Check sheet for the modelled part. Datum: model origin and axes. Units: mm. Round coordinates to 2 decimals unless told otherwise and drop trailing zeros. Order: outer loops, then holes, each group sorted by start corner. A loop starts at its lowest first (then second) coordinate and runs counter-clockwise, first axis right, second up. Notation, with made-up numbers: (75, 71.5) -> (121, 71.5) arc R13 ccw to (121, 93.5) -> close; hole circle Ø4 at (-34.5, 26). An arc over 180 degrees is marked (long way). Answer as CSV lines item,"result". Start each with the question number.
from build123d import *

# Parameters (mm, degrees)
SKETCH1_R           = 48.5
SKETCH1_R_2         = 4.7625
BOSS_EXTRUDE1_DEPTH = 10
CUT_EXTRUDE1_DEPTH  = 5000
SKETCH3_R           = 4.7625
CUT_EXTRUDE2_DEPTH  = 5000


with BuildPart() as part:
    # Sketch1 → Boss-Extrude1 (new body)
    with BuildSketch(Plane(origin=(0, 0, 0), x_dir=(1, 0, 0), z_dir=(0, 1, 0))):
        Polygon((205, 610), (-205, 610), (-305, 510), (-305, 100), (-205, 0), (205, 0), (305, 100), (305, 510), align=None)
        with Locations((-167.82128445, 168.589357775)):
            Circle(SKETCH1_R, mode=Mode.SUBTRACT)
        with Locations((-97, 168.589357775)):
            Circle(SKETCH1_R_2, mode=Mode.SUBTRACT)
        with Locations((97, 168.589357775)):
            Circle(SKETCH1_R_2, mode=Mode.SUBTRACT)
        with Locations((167.82128445, 168.589357775)):
            Circle(SKETCH1_R, mode=Mode.SUBTRACT)
        with Locations((-167.82128445, 441.410642225)):
            Circle(SKETCH1_R, mode=Mode.SUBTRACT)
        with Locations((-97, 441.410642225)):
            Circle(SKETCH1_R_2, mode=Mode.SUBTRACT)
        with Locations((97, 441.410642225)):
            Circle(SKETCH1_R_2, mode=Mode.SUBTRACT)
        with Locations((167.82128445, 441.410642225)):
            Circle(SKETCH1_R, mode=Mode.SUBTRACT)
    extrude(amount=BOSS_EXTRUDE1_DEPTH)

    # Sketch2 → Cut-Extrude1 (cut)
    with BuildSketch(Plane(origin=(0, 10, 0), x_dir=(1, 0, 0), z_dir=(0, 1, 0))):
        Polygon((-111, 69), (-180, 0), (180, 0), (111, 69), align=None)
    extrude(amount=-CUT_EXTRUDE1_DEPTH, mode=Mode.SUBTRACT)

    # Sketch3 → Cut-Extrude2 (cut)
    with BuildSketch(Plane(origin=(0, 10, 0), x_dir=(1, 0, 0), z_dir=(0, 1, 0))):
        with Locations((-205, 22.45771137)):
            Circle(SKETCH3_R)
        with Locations((205, 22.45771137)):
            Circle(SKETCH3_R)
        with Locations((-282.54228863, 100)):
            Circle(SKETCH3_R)
        with Locations((282.54228863, 100)):
            Circle(SKETCH3_R)
        with Locations((282.54228863, 510)):
            Circle(SKETCH3_R)
        with Locations((205, 587.54228863)):
            Circle(SKETCH3_R)
        with Locations((-205, 587.54228863)):
            Circle(SKETCH3_R)
        with Locations((-282.54228863, 510)):
            Circle(SKETCH3_R)
    extrude(amount=-CUT_EXTRUDE2_DEPTH, mode=Mode.SUBTRACT)


solid = part.part
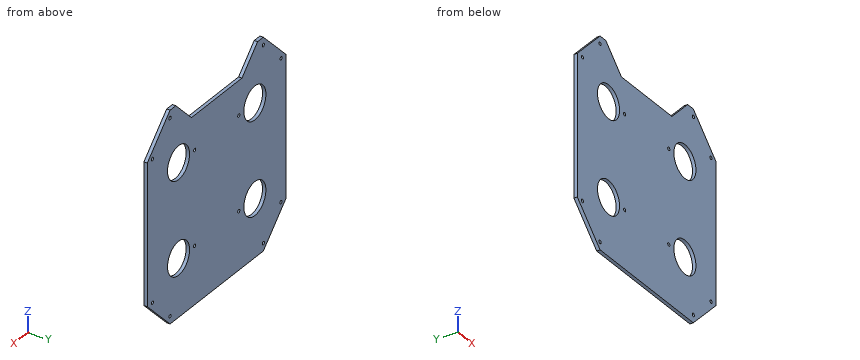
1) Depth check by flat-ended pin: pin 1 Ø1 at (x, y) = (-221.5, 7.5) entering from -Z; pin 2 Ø6 at (x, y) = (-146.5, 7) entering from +Z; pin 3 Ø2 at (x, y) = (-84.5, 6) entering from +Z. Enter the tip coordinate at first touch or a pass-through.
2) Section check B-B on y = 4.75. Count the separate pieces of the cut face and the enclosed holes in it, then the cut area to 3 significant figures.
3) Material ranges on line 1 along Z through (x, y) = (-97, 5.5); line 2 along X through (y, z) = (9, -428.5); line 3 along X through (y, z) = (9, -192.5), recorded low to high.
4) Section check C-C on x = 231.5. Record the cut outline in (y, z), then the cut area to 3 significant figures.
5) Section check D-D on x = -259. Record the cut outline in (y, z), then the cut area to 3 significant figures.
6) Section check A-A on x = -164.5. Record the cut outline in (y, z), then the cut area to 3 significant figures.
Solutions:
1,pin 1,"stops at z = -594"
1,pin 2,"stops at z = -30.5"
1,pin 3,"stops at z = -69"
2,separate pieces,"1"
2,enclosed holes,"16"
2,area,"302,000 mm^2"
3,line 1,"z = -610 to -446.17, -436.65 to -173.35, -163.83 to -69"
3,line 2,"x = -305 to -214.57, -121.07 to 121.07, 214.57 to 305"
3,line 3,"x = -305 to -210.02, -125.62 to 125.62, 210.02 to 305"
4,outline,"(0, -583.5) -> (10, -583.5) -> (10, -26.5) -> (0, -26.5) -> close"
4,area,"5,570 mm^2"
5,outline,"(0, -556) -> (10, -556) -> (10, -54) -> (0, -54) -> close"
5,area,"5,020 mm^2"
6,outline,"(0, -610) -> (10, -610) -> (10, -489.8) -> (0, -489.8) -> close; (0, -393.02) -> (10, -393.02) -> (10, -216.98) -> (0, -216.98) -> close; (0, -120.2) -> (10, -120.2) -> (10, -15.5) -> (0, -15.5) -> close"
6,area,"4,010 mm^2"
